Source: three-view drawing plus pictorial views. Frame: mm from the lowest corner of the part. A direction names the side the tool comes from. Give positions to 0.01 mm unless a question says otherwise; leave off trailing zeros. Order: outer loops, then holes, each group sorted by start corner. A loop starts at its lowest first (then second) coordinate and runs counter-clockwise, first axis right, second up. Notation, with made-up numbers: (-33, 71.5) -> (-23, 71.5) arc R23 cw to (-23, 99.5) -> close; hole circle Ø4 at (21.25, 58). An arc over 180 degrees is marked (long way). Answer in a Markdown table with one row per item. Add a question column.
Q1. Set-up query: the marked faces 1, 2 and 3. Return all of +Z, -Z, +X, -X, +Y, -Y with unobstructed straight access to the full face (end or side cutting, diameter ignored); none if empty.
Q2. Line query: line 1 along Z through (x, y) = (3.5, 21.5); line 2 along Y through (x, z) = (51, 32.5); line 3 along X through (y, z) = (4.5, 4). Output: solid intervals per line, ascending. Write a range as from..to.
Q3. Cut plane B-B on y = 21.75. Return the cut outline in (x, z).
Q4. Cut plane A-A on x = 10.5. Return the cut outline in (y, z).
Q5. Cut plane D-D on y = 3.25. Return the cut outline in (x, z).
Q6. Cut plane C-C on z = 6.5. Return the cut outline in (x, y), and give its area (3 significant figures).
Q7. Contact query for flat-ended pins moving along their axis: P1, Ø1.8, axis at x = 10.5, y = 24, coming from the -Z side; P2, Ø9.5, axis at x = 36.5, z = 14, coming from the -Y side; P3, Ø4, axis at y = 8.5, z = 26.5, coming from the -X side; P4, Ø5, axis at x = 20.5, y = 3, coming from the +Z side. Output: stop coordinate, or through.
Q8. Pull-direction query (Z, two-part tool) for the marked faces 4, 5, 6 and 7; classes: +Z half, -Z half, draft (parallel to the pull), parting line (faces both ways), or undercut.
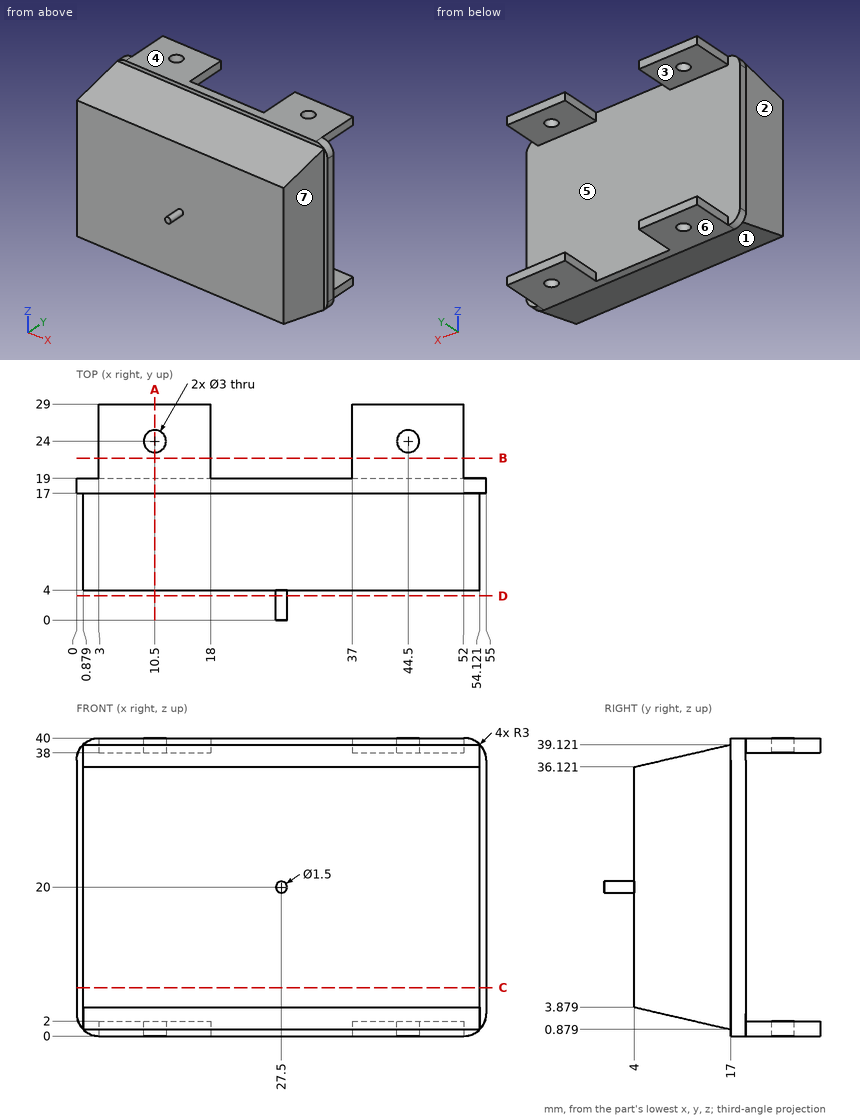
Completed:
| question | item | result |
|---|---|---|
| 1 | face 1 | -Z, +X, -X, -Y |
| 1 | face 2 | +Z, -Z, -X, -Y |
| 1 | face 3 | +X, -X, +Y |
| 2 | line 1 | z = 0..2, 38..40 |
| 2 | line 2 | y = 4..19 |
| 2 | line 3 | x = 0.88..54.12 |
| 3 | outline | (3, 0) -> (18, 0) -> (18, 2) -> (3, 2) -> close; (3, 38) -> (18, 38) -> (18, 40) -> (3, 40) -> close; (37, 0) -> (52, 0) -> (52, 2) -> (37, 2) -> close; (37, 38) -> (52, 38) -> (52, 40) -> (37, 40) -> close |
| 4 | outline | (4, 3.88) -> (17, 0.88) -> (17, 0) -> (22.5, 0) -> (22.5, 2) -> (19, 2) -> (19, 38) -> (22.5, 38) -> (22.5, 40) -> (17, 40) -> (17, 39.12) -> (4, 36.12) -> close; (25.5, 0) -> (29, 0) -> (29, 2) -> (25.5, 2) -> close; (25.5, 38) -> (29, 38) -> (29, 40) -> (25.5, 40) -> close |
| 5 | outline | circle Ø1.5 at (27.5, 20) |
| 6 | outline | (0, 17) -> (0.88, 17) -> (0.88, 4) -> (54.12, 4) -> (54.12, 17) -> (55, 17) -> (55, 19) -> (0, 19) -> close |
| 6 | area | 802 mm² |
| 7 | P1 | passes through |
| 7 | P2 | stops at y = 4 |
| 7 | P3 | stops at x = 0.88 |
| 7 | P4 | stops at z = 36.47 |
| 8 | face 4 | +Z half |
| 8 | face 5 | undercut |
| 8 | face 6 | -Z half |
| 8 | face 7 | draft |
